```python
from build123d import *

# Parameters (mm, degrees)
SKETCH_2_W      = 60
SKETCH_2_H      = 60
SKETCH_2_R      = 2
SKETCH_2_W_2    = 20
SKETCH_2_H_2    = 2
SKETCH_2_W_3    = 2
SKETCH_2_H_3    = 20
SKETCH_2_W_4    = 30
EXTRUDE_1_DEPTH = 2


with BuildPart() as part:
    # 草图2 → 凸台-拉伸1 (new body)
    # profile 1 of 4: a face of its own
    with BuildSketch(Plane.XY):
        with Locations((30, 30)):
            Rectangle(SKETCH_2_W, SKETCH_2_H)
        with Locations((25, 53)):
            Circle(SKETCH_2_R, mode=Mode.SUBTRACT)
        with Locations((35, 53)):
            Circle(SKETCH_2_R, mode=Mode.SUBTRACT)
        with Locations((30, 11)):
            Rectangle(SKETCH_2_W_2, SKETCH_2_H_2, mode=Mode.SUBTRACT)
        with Locations((30, 30)):
            Rectangle(SKETCH_2_W_3, SKETCH_2_H_3, mode=Mode.SUBTRACT)
    # profile 2 of 4: a face of its own
    with BuildSketch(Plane.XY):
        with Locations((30, 61)):
            Rectangle(SKETCH_2_W_4, SKETCH_2_H_2)
    # profile 3 of 4: a face of its own
    with BuildSketch(Plane.XY):
        with Locations((-1, 30)):
            Rectangle(SKETCH_2_W_3, SKETCH_2_H_3)
    # profile 4 of 4: a face of its own
    with BuildSketch(Plane.XY):
        with Locations((61, 30)):
            Rectangle(SKETCH_2_W_3, SKETCH_2_H_3)
    extrude(amount=EXTRUDE_1_DEPTH)


solid = part.part
```
Verification items for the finished model (mm, model axes). A direction names the side the tool comes from. Give positions to 0.01 mm unless a question says otherwise; leave off trailing zeros. Order: outer loops, then holes, each group sorted by start corner. A loop starts at its lowest first (then second) coordinate and runs counter-clockwise, first axis right, second up. Notation, with made-up numbers: M -4.75,86 L 24.25,86 A26 ccw 24.25,108 Z; hole C -35.75,41 d1. An arc over 180 degrees is marked long. Return JSON: item names as keys, results as strings. Group by question number.
1) Section check D-D on x = 35. Record the cut outline in (y, z).
2) Section check B-B on z = 0.7. Record the cut outline in (x, y).
3) Access from +Z, -Z, +X, -X, +Y, -Y to the whole of each face (thin tool, end or side, straight path). Record for faces 5 (the face through (0, 50, 1)), 6 (the face through (0, 10, 1)), 7 (the face through (30, 20, 1)).
4) Scan lines: line 1 (Y direction, x = 25, z = 1.35); line 2 (X direction, y = 24.5, z = 0.7); line 3 (Y direction, x = 38, z = 1.7). Record each from-to range of solid material in increasing order.
5) Section check A-A on y = 53. Record the cut outline in (x, z), and give its area (3 significant figures).
6) Section check C-C on y = 34. Record the cut outline in (x, z).
7) Mould release check, pull along X, two halves, no side actions. Record for faces 1 (the face through (-2, 30, 1)), 2 (the face through (31, 30, 1)), 3 (the face through (60, 10, 1)), 4 (the face through (30, 0, 1)): pulls with the +X half, pulls with the -X half, needs draft (parallel to the pull), parting line crosses it, or undercut.
8) Go/stop test with flat-tipped pins: pin 1 Ø1 at (y, z) = (46.5, 1) entering from -X; pin 2 Ø0.6 at (x, z) = (53, 1.5) entering from +Y; pin 3 Ø0.6 at (x, z) = (-1, 0.5) entering from -Y; pin 4 Ø4.5 at (x, y) = (25, 53) entering from +Z. Record where each tip stops, or that it passes through.
Answer block:
{
 "1": {"outline": "M 0,0 L 10,0 L 10,2 L 0,2 Z; M 12,0 L 51,0 L 51,2 L 12,2 Z; M 55,0 L 62,0 L 62,2 L 55,2 Z"},
 "2": {"outline": "M -2,20 L 0,20 L 0,0 L 60,0 L 60,20 L 62,20 L 62,40 L 60,40 L 60,60 L 45,60 L 45,62 L 15,62 L 15,60 L 0,60 L 0,40 L -2,40 Z; hole M 20,10 L 40,10 L 40,12 L 20,12 Z; hole C 25,53 d4; hole M 29,20 L 31,20 L 31,40 L 29,40 Z; hole C 35,53 d4"},
 "3": {"face 5": "+Z, -Z, -X, +Y", "face 6": "+Z, -Z, -X, -Y", "face 7": "+Z, -Z"},
 "4": {"line 1": "y = 0 to 10, 12 to 51, 55 to 62", "line 2": "x = -2 to 29, 31 to 62", "line 3": "y = 0 to 10, 12 to 62"},
 "5": {"outline": "M 0,0 L 23,0 L 23,2 L 0,2 Z; M 27,0 L 33,0 L 33,2 L 27,2 Z; M 37,0 L 60,0 L 60,2 L 37,2 Z", "area": "104 mm^2"},
 "6": {"outline": "M -2,0 L 29,0 L 29,2 L -2,2 Z; M 31,0 L 62,0 L 62,2 L 31,2 Z"},
 "7": {"face 1": "pulls with the -X half", "face 2": "undercut", "face 3": "pulls with the +X half", "face 4": "needs draft"},
 "8": {"pin 1": "stops at x = 0", "pin 2": "stops at y = 60", "pin 3": "stops at y = 20", "pin 4": "stops at z = 2"}
}
